Design review of the part built by this model. Coordinates are the model's own, in mm. A direction names the side the tool comes from. Coordinates: 2 decimals unless noted, no trailing zeros. Loops run counter-clockwise (first coordinate to the right, second up) from the corner with the lowest first, then second, coordinate; pieces in that order, holes last. Notation, with made-up numbers: (75, 4.5) -> (94, 4.5) arc R18 cw to (94, 28.5) -> close; hole circle Ø4 at (64, 13.5). An arc over 180 degrees is marked (long way). One line per item, written item: value. Start each with the question number.
1. Draft analysis for pull direction Z (two halves, no side actions). For faces 1 (the flat face through (-97.5, 2, -1)), 2 (the flat face through (-1, 2, 72.5)), 3 (the flat face through (-94.5, 3, 65)), state which applies: pulls with the +Z half, pulls with the -Z half, needs draft (parallel to the pull), parting line crosses it, or undercut.
2. For probe 1 along Z at (x, y) = (-14, 1); probe 2 along X at (y, z) = (15, 0); probe 3 along Y at (x, z) = (88, -29), list the stretches that pass through material, from the lowest coordinate up.
3. Add section A-A on x = -24. Write out the cut boundary in (y, z), plus the area to 3 significant figures.
4. Add section C-C on y = 17. Write out the cut boundary in (x, z), plus the area to 3 significant figures.
5. Insertion check: pin 1 (5 mm diameter, centred on x = -33, z = -40, fed in from +Y); pin 2 (2.5 mm diameter, centred on x = 89, y = 1.5, fed in from +Z); pin 3 (1.5 mm diameter, centred on x = 89.5, y = 3.5, fed in from -Z). Each pin has a flat end and moves straight along its axis. Give the tip position at first contact, or say it passes through.
6. Machinability: for faces 4 (the flat face through (82.5, 3, -27)), 5 (the flat face through (3, 24.5, -14)), which of the approach directions +Z, -Z, +X, -X, +Y, -Y give a long, thin tool a straight path to every point of the face, cutting with its end or side? Answer none if there is none.
7. Add section B-B on z = 21.5. Write out the cut boundary in (x, y), plus the area to 3 significant figures.
8. Add section D-D on x = 0. Write out the cut boundary in (y, z).
```python
from build123d import *

# Parameters (mm, degrees)
BOSS_EXTRUDE2_DEPTH = 5
SKETCH5_W           = 5
SKETCH5_H           = 45
SKETCH5_W_2         = 70
SKETCH5_H_2         = 5
CUT_EXTRUDE5_DEPTH  = 6
BOSS_EXTRUDE3_DEPTH = 19.5
FILLET1_R           = 10
CUT_EXTRUDE6_DEPTH  = 5


with BuildPart() as part:
    # Sketch4 → Boss-Extrude2 (new body)
    with BuildSketch(Plane(origin=(0, 0, 0), x_dir=(1, 0, 0), z_dir=(0, 1, 0))):
        Polygon((0, 0), (-97.5, 72.5), (-97.5, -72.5), align=None)
        Polygon((0, 0), (-97.5, -72.5), (97.5, -72.5), align=None)
        Polygon((97.5, 72.5), (-97.5, 72.5), (0, 0), align=None)
        Polygon((97.5, -72.5), (97.5, 72.5), (0, 0), align=None)
    extrude(amount=BOSS_EXTRUDE2_DEPTH)

    # Sketch5 → Cut-Extrude5 (cut, through all)
    with BuildSketch(Plane(origin=(0, 5, 0), x_dir=(1, 0, 0), z_dir=(0, 1, 0))):
        with Locations((-85, 27.5)):
            Rectangle(SKETCH5_W, SKETCH5_H)
        with Locations((-85, -27.5)):
            Rectangle(SKETCH5_W, SKETCH5_H)
        with Locations((-40, -60)):
            Rectangle(SKETCH5_W_2, SKETCH5_H_2)
        with Locations((40, -60)):
            Rectangle(SKETCH5_W_2, SKETCH5_H_2)
        with Locations((85, -27.5)):
            Rectangle(SKETCH5_W, SKETCH5_H)
        with Locations((85, 27.5)):
            Rectangle(SKETCH5_W, SKETCH5_H)
        with Locations((40, 60)):
            Rectangle(SKETCH5_W_2, SKETCH5_H_2)
        with Locations((-40, 60)):
            Rectangle(SKETCH5_W_2, SKETCH5_H_2)
    extrude(amount=-CUT_EXTRUDE5_DEPTH, mode=Mode.SUBTRACT)

    # Sketch6 → Boss-Extrude3 (add)
    with BuildSketch(Plane(origin=(0, 5, 0), x_dir=(1, 0, 0), z_dir=(0, 1, 0))):
        with BuildLine():
            ThreePointArc((15.9, 0), (-5.30377301, 14.989329267), (-12.361634196, -10))
            Line((-12.361634196, -10), (-9.654532614, -10))
            ThreePointArc((-9.654532614, -10), (-5.431942409, 12.794686462), (13.9, 0))
            ThreePointArc((13.9, 0), (12.794686462, -5.431942409), (9.654532614, -10))
            Line((9.654532614, -10), (12.361634196, -10))
            ThreePointArc((12.361634196, -10), (14.989329267, -5.30377301), (15.9, 0))
        make_face()
    extrude(amount=BOSS_EXTRUDE3_DEPTH)

    # Fillet1
    fillet1_edges = [part.edges().sort_by_distance(p)[0] for p in [
        (-97.5, 2.5, 72.5),
        (-97.5, 2.5, -72.5),
        (97.5, 2.5, -72.5),
        (97.5, 2.5, 72.5),
    ]]
    fillet(fillet1_edges, radius=FILLET1_R)

    # Sketch7 → Cut-Extrude6 (cut)
    with BuildSketch(Plane(origin=(0, 5, 0), x_dir=(1, 0, 0), z_dir=(0, 1, 0))):
        Polygon((-86.5, 69.5), (-94.5, 69.5), (-86.5, 63.616402116), align=None)
        Polygon((-94.5, 69.5), (-94.5, 61.5), (-86.5, 61.5), (-86.5, 63.616402116), align=None)
        Polygon((-86.5, -61.5), (-94.5, -61.5), (-94.5, -69.5), (-86.5, -63.616402116), align=None)
        Polygon((-86.5, -63.616402116), (-94.5, -69.5), (-86.5, -69.5), align=None)
        Polygon((86.5, -63.616402116), (86.5, -69.5), (94.5, -69.5), align=None)
        Polygon((86.5, -61.5), (86.5, -63.616402116), (94.5, -69.5), (94.5, -61.5), align=None)
        Polygon((86.5, 69.5), (86.5, 63.616402116), (94.5, 69.5), align=None)
        Polygon((94.5, 69.5), (86.5, 63.616402116), (86.5, 61.5), (94.5, 61.5), align=None)
    extrude(amount=-CUT_EXTRUDE6_DEPTH, mode=Mode.SUBTRACT)


solid = part.part
```
Worked answers:
1. face 1: needs draft
1. face 2: pulls with the +Z half
1. face 3: undercut
2. probe 1: z = -72.5 to -62.5, -57.5 to 57.5, 62.5 to 72.5
2. probe 2: x = -15.9 to -13.9, 13.9 to 15.9
2. probe 3: y = 0 to 5
3. outline: (0, -72.5) -> (5, -72.5) -> (5, -62.5) -> (0, -62.5) -> close; (0, -57.5) -> (5, -57.5) -> (5, 57.5) -> (0, 57.5) -> close; (0, 62.5) -> (5, 62.5) -> (5, 72.5) -> (0, 72.5) -> close
3. area: 675 mm²
4. outline: (-12.36, 10) arc R15.9 ccw (long way) to (12.36, 10) -> (9.65, 10) arc R13.9 cw (long way) to (-9.65, 10) -> close
4. area: 138 mm²
5. pin 1: stops at y = 5
5. pin 2: stops at z = 72.5
5. pin 3: stops at z = -72.42
6. face 4: +Y, -Y
6. face 5: +Z, -Z, +X, -X, +Y
7. outline: (-97.5, 0) -> (-87.5, 0) -> (-87.5, 5) -> (-97.5, 5) -> close; (-82.5, 0) -> (82.5, 0) -> (82.5, 5) -> (-82.5, 5) -> close; (87.5, 0) -> (97.5, 0) -> (97.5, 5) -> (87.5, 5) -> close
7. area: 925 mm²
8. outline: (0, -72.5) -> (5, -72.5) -> (5, -15.9) -> (24.5, -15.9) -> (24.5, -13.9) -> (5, -13.9) -> (5, 72.5) -> (0, 72.5) -> close
